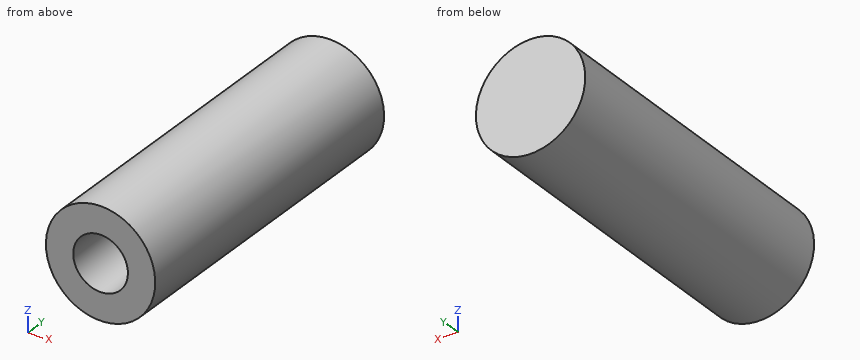
```python
from build123d import *

# Parameters (mm, degrees)
SKETCH2_R           = 5
BOSS_EXTRUDE1_DEPTH = 30
SKETCH3_R           = 2.5
CUT_EXTRUDE1_DEPTH  = 10
CUT_EXTRUDE2_DEPTH  = 10


with BuildPart() as part:
    # Sketch2 → Boss-Extrude1 (new body)
    with BuildSketch(Plane(origin=(0, 0, 0), x_dir=(1, 0, 0), z_dir=(0, 1, 0))):
        with Locations(Location((0, 0, 0), (0, 0, 270))):
            Circle(SKETCH2_R)
    extrude(amount=BOSS_EXTRUDE1_DEPTH)

    # Sketch3 → Cut-Extrude1 (cut)
    with BuildSketch(Plane(origin=(0, 0, 0), x_dir=(-1, 0, 0), z_dir=(0, -1, 0))):
        with Locations(Location((0, 0, 0), (0, 0, 90))):
            Circle(SKETCH3_R)
    extrude(amount=-CUT_EXTRUDE1_DEPTH, mode=Mode.SUBTRACT)

    # Sketch4 → Cut-Extrude2 (cut)
    with BuildSketch(Plane.XZ.offset(-10)):
        with BuildLine():
            Line((2, 1.5), (2, -1.5))
            ThreePointArc((2, -1.5), (-2.5, 0), (2, 1.5))
        make_face()
    extrude(amount=-CUT_EXTRUDE2_DEPTH, mode=Mode.SUBTRACT)


solid = part.part
```
Input: part model. Units: mm. Frame: model coordinates. Give positions to 0.01 mm unless a question says otherwise; leave off trailing zeros. Loops run counter-clockwise (first coordinate to the right, second up) from the corner with the lowest first, then second, coordinate; pieces in that order, holes last. Notation, with made-up numbers: (61, 74) -> (89, 74) arc R29 ccw to (89, 108) -> close; hole circle Ø11 at (15.25, -25). An arc over 180 degrees is marked (long way). Use a Markdown table: item, result.
Q1. Section query C-C, the plane y = 14. Return the cut outline in (x, z), plus the area to 3 significant figures.
Entries:
| item | result |
|---|---|
| outline | circle Ø10 at (0, 0); hole (2, -1.5) -> (2, 1.5) arc R2.5 ccw (long way) to start |
| area | 59.9 mm² |
Q2. Section query B-B, the plane z = 0. Return the cut outline in (x, y), plus the area to 3 significant figures.
Entries:
| item | result |
|---|---|
| outline | (-5, 0) -> (-2.5, 0) -> (-2.5, 20) -> (2, 20) -> (2, 10) -> (2.5, 10) -> (2.5, 0) -> (5, 0) -> (5, 30) -> (-5, 30) -> close |
| area | 205 mm² |
Q3. Section query A-A, the plane x = 0. Return the cut outline in (y, z).
Entries:
| item | result |
|---|---|
| outline | (0, -5) -> (30, -5) -> (30, 5) -> (0, 5) -> (0, 2.5) -> (20, 2.5) -> (20, -2.5) -> (0, -2.5) -> close |
Q4. First-contact query: P1, Ø5, axis at y = 6, z = -3, coming from the -X side; P2, Ø4, axis at x = -2.5, y = 21.5, coming from the -Z side; P3, Ø1.3, axis at x = 0.5, z = 0, coming from the -Y side. Flat tips, straight axial feed; report the tip coordinate or a pass-through.
Entries:
| item | result |
|---|---|
| P1 | stops at x = -4.97 |
| P2 | stops at z = -4.97 |
| P3 | stops at y = 20 |
Q5. Ray query, probe 1 along X at (y, z) = (4, 0); probe 2 along X at (y, z) = (14.25, 0); probe 3 along Y at (x, z) = (-1.5, 0.75). Return the intervals inside material, ascending. Write a range as from..to.
Entries:
| item | result |
|---|---|
| probe 1 | x = -5..-2.5, 2.5..5 |
| probe 2 | x = -5..-2.5, 2..5 |
| probe 3 | y = 20..30 |
Q6. Section query D-D, the plane y = 28. Return the cut outline in (x, z).
Entries:
| item | result |
|---|---|
| outline | circle Ø10 at (0, 0) |
